The model under review builds one solid part; all positions refer to its coordinate system, in mm. A direction names the side the tool comes from. Round coordinates to 2 decimals unless told otherwise and drop trailing zeros. Write each loop counter-clockwise with the first axis right and the second up, starting at its lowest first coordinate (ties: lowest second). Pieces come first, ordered by that corner, then holes. Notation, with made-up numbers: M 81.5,80.5 L 115.5,80.5 A33 cw 115.5,111.5 Z; hole C -15,83.5 d3. An arc over 180 degrees is marked long. One line per item, written item: value. Start each with the question number.
1) Take a section at D-D, the plane y = 6. Write out the cut boundary in (x, z).
2) Mouldability with a two-part tool opening along Z and no side actions: class faces 4 (the face through (69.26, -17.02, 7.83)), 5 (the face through (72, 36, 8)), 6 (the face through (70.99, 11, 2.73)) as +Z half, -Z half, draft (parallel to the pull), parting line (faces both ways), or undercut.
3) Take a section at A-A, the plane z = 7.5. Write out the cut boundary in (x, y).
4) Take a section at B-B, the plane x = 18. Write out the cut boundary in (y, z), and give its area (3 significant figures).
5) Wall thickness on probe 1 along Y at (x, z) = (69.3, 7.5); probe 2 along Y at (x, z) = (18, 7.5); probe 3 along Y at (x, z) = (4.5, 7): over which ranges is each line inside the solid? List them lowest first.
6) For P1, Ø5, axis at x = 60.5, z = 14, coming from the -Y side; P2, Ø22.5, axis at x = 40, y = 21.5, coming from the +Z side; P3, Ø8, axis at x = 48.5, y = 50.5, coming from the -Z side; P4, Ø5, axis at x = 20, y = 29.5, coming from the -Z side, all flat-tipped, find the tip position at first contact; note any pin that passes through.
7) Take a section at C-C, the plane y = 64.5. Write out the cut boundary in (x, z), and give its area (3 significant figures).
8) Tool access review of faces 1 (the face through (68.5, -14, 8)), 2 (the face through (70.986, 39.716, 4.812)), 3 (the face through (68.5, 59, 8)): name each direction out of +Z, -Z, +X, -X, +Y, -Y from which nothing blocks a thin tool from reaching the whole face with its end or side.
from build123d import *

# Parameters (mm, degrees)
SKETCH1_W           = 70
SKETCH1_H           = 45
SKETCH1_R           = 3
BOSS_EXTRUDE1_DEPTH = 15
SKETCH2_R           = 2.5
BOSS_EXTRUDE2_DEPTH = 1.5
SKETCH3_R           = 5
BOSS_EXTRUDE3_DEPTH = 2


with BuildPart() as part:
    # Sketch1 → Boss-Extrude1 (new body)
    with BuildSketch(Plane.XY):
        with Locations((35, 22.5)):
            Rectangle(SKETCH1_W, SKETCH1_H)
        with Locations((18, 22.5)):
            Circle(SKETCH1_R, mode=Mode.SUBTRACT)
    extrude(amount=BOSS_EXTRUDE1_DEPTH)

    # Sketch2 → Boss-Extrude2 (add)
    with BuildSketch(Plane(origin=(70, 0, 0), x_dir=(0, 0, -1), z_dir=(1, 0, 0))):
        Polygon((-1, 42.953382973), (-1, 47), (1.5, 47), (1.5, 72.5), (-16.5, 72.5), (-16.5, 47), (-14, 47), (-14, 42.953382973), align=None)
        with Locations((-7.5, 64.5)):
            Circle(SKETCH2_R, mode=Mode.SUBTRACT)
        Polygon((-14, 2.046617027), (-14, -2), (-16.5, -2), (-16.5, -27.5), (1.5, -27.5), (1.5, -2), (-1, -2), (-1, 2.046617027), align=None)
        with Locations((-7.5, -19.5)):
            Circle(SKETCH2_R, mode=Mode.SUBTRACT)
    extrude(amount=-BOSS_EXTRUDE2_DEPTH)

    # Sketch3 → Boss-Extrude3 (add)
    with BuildSketch(Plane(origin=(70, 0, 0), x_dir=(0, 0, -1), z_dir=(1, 0, 0))):
        with Locations((-7.5, 35.5)):
            Circle(SKETCH3_R)
        with Locations((-7.5, 9.5)):
            Circle(SKETCH3_R)
    extrude(amount=BOSS_EXTRUDE3_DEPTH)


solid = part.part
Checked values:
1. outline: M 0,0 L 70,0 L 70,3.93 L 72,3.93 L 72,11.07 L 70,11.07 L 70,15 L 0,15 Z
2. face 4: undercut
2. face 5: draft
2. face 6: parting line
3. outline: M 0,0 L 68.5,0 L 68.5,-17 L 70,-17 L 70,4.5 L 72,4.5 L 72,14.5 L 70,14.5 L 70,30.5 L 72,30.5 L 72,40.5 L 70,40.5 L 70,62 L 68.5,62 L 68.5,45 L 0,45 Z; M 68.5,-27.5 L 70,-27.5 L 70,-22 L 68.5,-22 Z; M 68.5,67 L 70,67 L 70,72.5 L 68.5,72.5 Z; hole C 18,22.5 d6
4. outline: M 0,0 L 19.5,0 L 19.5,15 L 0,15 Z; M 25.5,0 L 45,0 L 45,15 L 25.5,15 Z
4. area: 585 mm2
5. probe 1: y = -27.5 to -22, -17 to 62, 67 to 72.5
5. probe 2: y = 0 to 19.5, 25.5 to 45
5. probe 3: y = 0 to 45
6. P1: stops at y = 0
6. P2: stops at z = 15
6. P3: passes through
6. P4: stops at z = 0
7. outline: M 68.5,-1.5 L 70,-1.5 L 70,5 L 68.5,5 Z; M 68.5,10 L 70,10 L 70,16.5 L 68.5,16.5 Z
7. area: 19.5 mm2
8. face 1: +Z, -Z, -X, -Y
8. face 2: +X
8. face 3: +Z, -Z, -X, +Y
